Input: part model. Units: mm. Frame: model coordinates. Give positions to 0.01 mm unless a question says otherwise; leave off trailing zeros. Order: outer loops, then holes, each group sorted by start corner. A loop starts at its lowest first (then second) coordinate and runs counter-clockwise, first axis right, second up. Notation, with made-up numbers: (-4.5, 87) - (44.5, 87) arc R13 ccw to (44.5, 100) - close; hole circle Ø2 at (31, -22.75). An arc over 180 degrees is marked (long way). Answer in a Markdown table with one row per item. Add a question column.
1. Section query B-B on x = 0. Return loops of the section in (y, z), and give its area (4 significant figures).
2. Section query A-A on y = -100. Return loops of the section in (x, z), and give its area (4 significant figures).
3. Section query C-C on y = 0. Return loops of the section in (x, z).
4. Ray query, line 1 (Y direction, x = -60.5, z = 0.9); line 2 (Y direction, x = 0, z = 0.85); line 3 (X direction, y = 52, z = 0.65). Return the intervals inside material, ascending. Write a range as [from, to].
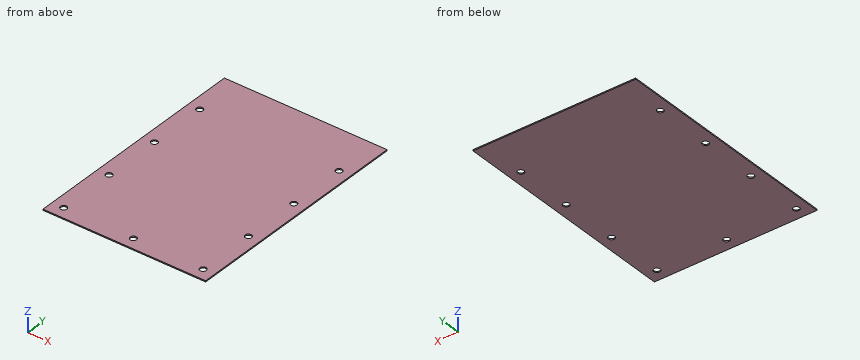
```python
from build123d import *

# Parameters (mm, degrees)
SKETCH_1_W          = 140
SKETCH_1_H          = 220
EXTRUDE_1_DEPTH     = 1
HOLE_WIZARD_M5_1_D  = 5.5
SKETCH_4_W          = 140
SKETCH_4_H          = 20
CUT_EXTRUDE_1_DEPTH = 10


with BuildPart() as part:
    # 스케치1 → 보스-돌출1 (new body)
    with BuildSketch(Plane.XY):
        Rectangle(SKETCH_1_W, SKETCH_1_H)
    extrude(amount=EXTRUDE_1_DEPTH)

    # M5 여유 구멍1 (through all)
    with Locations(Plane(origin=(0, 0, 0), x_dir=(-1, 0, 0), z_dir=(0, 0, -1))):
        with Locations((-60, 100), (0, 100), (60, 100), (60, 50), (60, -50), (60, 0), (60, -100), (-60, 50), (-60, -50), (-60, 0), (-60, -100), (0, -100)):
            Hole(HOLE_WIZARD_M5_1_D / 2)

    # 스케치4 → 컷-돌출1 (cut)
    with BuildSketch(Plane(origin=(0, 0, 0), x_dir=(-1, 0, 0), z_dir=(0, 0, -1))):
        with Locations((0, 100)):
            Rectangle(SKETCH_4_W, SKETCH_4_H)
    extrude(amount=-CUT_EXTRUDE_1_DEPTH, mode=Mode.SUBTRACT)


solid = part.part
```
Answer:
| question | item | result |
|---|---|---|
| 1 | outline | (-110, 0) - (-102.75, 0) - (-102.75, 1) - (-110, 1) - close; (-97.25, 0) - (90, 0) - (90, 1) - (-97.25, 1) - close |
| 1 | area | 194.5 mm² |
| 2 | outline | (-70, 0) - (-62.75, 0) - (-62.75, 1) - (-70, 1) - close; (-57.25, 0) - (-2.75, 0) - (-2.75, 1) - (-57.25, 1) - close; (2.75, 0) - (57.25, 0) - (57.25, 1) - (2.75, 1) - close; (62.75, 0) - (70, 0) - (70, 1) - (62.75, 1) - close |
| 2 | area | 123.5 mm² |
| 3 | outline | (-70, 0) - (-62.75, 0) - (-62.75, 1) - (-70, 1) - close; (-57.25, 0) - (57.25, 0) - (57.25, 1) - (-57.25, 1) - close; (62.75, 0) - (70, 0) - (70, 1) - (62.75, 1) - close |
| 4 | line 1 | y = [-110, -102.7], [-97.3, -52.7], [-47.3, -2.7], [2.7, 47.3], [52.7, 90] |
| 4 | line 2 | y = [-110, -102.75], [-97.25, 90] |
| 4 | line 3 | x = [-70, -61.89], [-58.11, 58.11], [61.89, 70] |
